Could you check a few things on this model? Use its own coordinates, in mm. Face numbers are marked on the shaded views. A direction names the side the tool comes from. Coordinates: 2 decimals unless noted, no trailing zeros. Write each loop counter-clockwise with the first axis right and the second up, starting at its lowest first coordinate (ties: lowest second). Pieces come first, ordered by that corner, then holes. Notation, with made-up numbers: (88.5, 33.25) - (137.5, 33.25) arc R32 cw to (137.5, 66.25) - close; hole circle Ø10 at (73, 77.5). An arc over 180 degrees is marked (long way). Answer as a JSON object with one key per item and string values. Group by question number.
1) If we section it at A-A (x = 57): Write out the boundary of the cut face in (y, z).
2) If we section it at D-D (x = 85): Write out the boundary of the cut face in (y, z).
3) Please list where these lines run through material, in increasing order: line 1 along X through (y, z) = (103.5, -68.5); line 2 along Z through (x, y) = (31.5, 13); line 3 along X through (y, z) = (40, 1).
4) If we section it at C-C (y = 15): Write out the boundary of the cut face in (x, z).
5) We'd pull the mould along X, two halves only. Please class the marked faces 3, 4, 5 and 6: released by +X, released by -X, zero draft, split by the parting line, or undercut.
6) If we section it at B-B (z = -37.5): Write out the boundary of the cut face in (x, y), plus the area to 3 significant figures.
7) Will these pins go through, and if not, where does the flat tip stop? pin 1 Ø3 at (x, z) = (44, -60) entering from +Y; pin 2 Ø3 at (x, y) = (28.5, 103) entering from +Z; pin 3 Ø9 at (x, z) = (62.5, -109) entering from +Y.
8) On a 3-axis mill with a long thin cutter (end or side, diameter ignored), from which of +Z, -Z, +X, -X, +Y, -Y can I reach the whole of each face in a straight line? I mean the marked faces 1 and 2. Say none if no direction works.
```python
from build123d import *

# Parameters (mm, degrees)
CROQUIS1_W                 = 120
CROQUIS1_H                 = 120
SALIENTE_EXTRUIR1_DEPTH    = 120
CORTAR_EXTRUIR1_DEPTH      = 120
CORTAR_EXTRUIR1_DEPTH_BACK = 120
CROQUIS3_R                 = 20
CORTAR_EXTRUIR2_DEPTH      = 120
CROQUIS4_W                 = 120
CROQUIS4_H                 = 120
SALIENTE_EXTRUIR2_DEPTH    = 3
CROQUIS4_3_W               = 98
CROQUIS4_3_H               = 8
CROQUIS4_3_W_2             = 8
CROQUIS4_3_H_2             = 98
SALIENTE_EXTRUIR3_DEPTH    = 8


with BuildPart() as part:
    # Croquis1 → Saliente-Extruir1 (new body)
    with BuildSketch(Plane(origin=(0, 0, 0), x_dir=(1, 0, 0), z_dir=(0, 1, 0))):
        with Locations((57, 57)):
            Rectangle(CROQUIS1_W, CROQUIS1_H)
        Polygon((8, 0), (106, 0), (106, 8), (114, 8), (114, 106), (106, 106), (106, 114), (8, 114), (8, 106), (0, 106), (0, 8), (8, 8), align=None, mode=Mode.SUBTRACT)
    extrude(amount=SALIENTE_EXTRUIR1_DEPTH)

    # Croquis2 → Cortar-Extruir1 (cut, two sides: drawn at the far end of the back side and taken through both)
    with BuildSketch(Plane(origin=(0, 0, 0), x_dir=(0, 0, -1), z_dir=(1, 0, 0)).offset(-CORTAR_EXTRUIR1_DEPTH_BACK)):
        Polygon((117, 120), (-3, 80), (-3, 120), align=None)
    extrude(amount=CORTAR_EXTRUIR1_DEPTH + CORTAR_EXTRUIR1_DEPTH_BACK, mode=Mode.SUBTRACT)

    # Croquis3 → Cortar-Extruir2 (cut)
    with BuildSketch(Plane.XY):
        with Locations(Location((57, 40, 0), (0, 0, 180))):
            Circle(CROQUIS3_R)
    extrude(amount=CORTAR_EXTRUIR2_DEPTH, mode=Mode.SUBTRACT)

    # Croquis4 → Saliente-Extruir2 (add)
    with BuildSketch(Plane(origin=(0, 0, 0), x_dir=(1, 0, 0), z_dir=(0, 1, 0))):
        with Locations((57, 57)):
            Rectangle(CROQUIS4_W, CROQUIS4_H)
    extrude(amount=-SALIENTE_EXTRUIR2_DEPTH)

    # Croquis4_3 → Saliente-Extruir3 (add)
    with BuildSketch(Plane(origin=(0, 0, 0), x_dir=(1, 0, 0), z_dir=(0, 1, 0))):
        with Locations((57, 110)):
            Rectangle(CROQUIS4_3_W, CROQUIS4_3_H)
        with Locations((110, 57)):
            Rectangle(CROQUIS4_3_W_2, CROQUIS4_3_H_2)
        with Locations((57, 4)):
            Rectangle(CROQUIS4_3_W, CROQUIS4_3_H)
        with Locations((4, 57)):
            Rectangle(CROQUIS4_3_W_2, CROQUIS4_3_H_2)
    extrude(amount=SALIENTE_EXTRUIR3_DEPTH)


solid = part.part
```
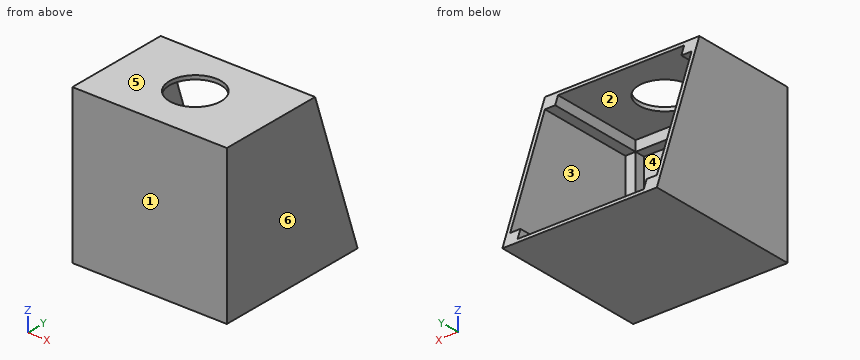
Here are the results:
{
 "1": {"outline": "(-3, -117) - (120, -117) - (119, -114) - (8, -114) - (8, -106) - (0, -106) - (0, -8) - (8, -8) - (8, 0) - (20, 0) - (20, 3) - (-3, 3) - close; (60, 0) - (81, 0) - (80, 3) - (60, 3) - close"},
 "2": {"outline": "(-3, -117) - (120, -117) - (119, -114) - (8, -114) - (8, -106) - (0, -106) - (0, -8) - (8, -8) - (8, 0) - (81, 0) - (80, 3) - (-3, 3) - close"},
 "3": {"line 1": "x = -3 to 0, 114 to 117", "line 2": "z = -117 to -114, 0 to 3", "line 3": "x = -3 to 37, 77 to 117"},
 "4": {"outline": "(-3, -117) - (117, -117) - (117, 3) - (-3, 3) - close; hole (0, -106) - (8, -106) - (8, -114) - (106, -114) - (106, -106) - (114, -106) - (114, -8) - (106, -8) - (106, 0) - (8, 0) - (8, -8) - (0, -8) - close"},
 "5": {"face 3": "undercut", "face 4": "undercut", "face 5": "zero draft", "face 6": "released by +X"},
 "6": {"outline": "(-3, -3) - (117, -3) - (117, 93.5) - (114, 93.5) - (114, 8) - (106, 8) - (106, 0) - (8, 0) - (8, 8) - (0, 8) - (0, 93.5) - (-3, 93.5) - close", "area": "1,050 mm²"},
 "7": {"pin 1": "stops at y = 0", "pin 2": "stops at z = -114", "pin 3": "stops at y = 8"},
 "8": {"face 1": "+Z, -Z, +X, -X, -Y", "face 2": "+Y"}
}
